The model under review builds one solid part; all positions refer to its coordinate system, in mm. A direction names the side the tool comes from. Round coordinates to 2 decimals unless told otherwise and drop trailing zeros. Write each loop counter-clockwise with the first axis right and the second up, starting at its lowest first coordinate (ties: lowest second). Pieces come first, ordered by that corner, then holes. Notation, with made-up numbers: (45, 88) - (80, 88) arc R11 ccw to (80, 97) - close; hole circle Ø10 at (37.25, 76). An arc over 180 degrees is marked (long way). Write each question's results on one line, items separated by ' | '.
```python
from build123d import *

# Parameters (mm, degrees)
F1_DEPTH      = 8
F1_DEPTH_BACK = 15
F0_R          = 3
F2_DEPTH      = 5
F3_R          = 2
F4_DEPTH      = 25


with BuildPart() as f1:
    # F0 (on Top) → F1 (new body, two sides)
    with BuildSketch(Plane.XY) as f1_sk:
        with BuildLine():
            Line((0, -25), (-25, 0))
            ThreePointArc((-25, 0), (-17.67767, -17.67767), (0, -25))
        make_face()
    extrude(amount=F1_DEPTH)
    extrude(f1_sk.sketch, amount=-F1_DEPTH_BACK)

    # F0 (on Top) → F2 (join)
    with BuildSketch(Plane.XY):
        with BuildLine():
            Line((-25, 0), (-30, 0))
            Line((-30, 0), (-30, -30))
            Line((-30, -30), (0, -30))
            Line((0, -30), (0, -25))
            ThreePointArc((0, -25), (-17.67767, -17.67767), (-25, 0))
        make_face()
        with Locations((-21.9205, -21.92012)):
            Circle(F0_R, mode=Mode.SUBTRACT)
    extrude(amount=F2_DEPTH)

    # F3 (on face) → F4 (cut)
    with BuildSketch(Plane(origin=(-12.5, -12.5, 0), x_dir=(-0.707107, 0.707107, 0), z_dir=(0.707107, 0.707107, 0))):
        with Locations((0, -9)):
            Circle(F3_R)
    extrude(amount=-F4_DEPTH, mode=Mode.SUBTRACT)


solid = f1.part
```
Q1. We need section D-D (x = -7). State the section outline as (y, z) points.
Evaluation:
outline: (-30, 0) - (-24, 0) - (-24, -15) - (-18, -15) - (-18, 8) - (-24, 8) - (-24, 5) - (-30, 5) - close
Q2. We need section C-C (z = -8). State the section outline as (x, y) points, plus the area to 3 significant figures.
Evaluation:
outline: (-25, 0) arc R25 ccw to (-18.86, -16.41) - (-13.72, -11.28) - close; (-16.41, -18.86) arc R25 ccw to (0, -25) - (-11.28, -13.72) - close | area: 153 mm^2
Q3. Insertion check: P1, Ø1, axis at x = -7.5, z = -12.5, coming from the +Y side; P2, Ø2, axis at y = -4.5, z = -3.5, coming from the -X side; P3, Ø1.5, axis at x = -4, z = -11.5, coming from the +Y side. Each pin has a flat end and moves straight along its axis. Give the tip position at first contact, or say it passes through.
Evaluation:
P1: stops at y = -17 | P2: stops at x = -24.75 | P3: stops at y = -20.25
Q4. Tool access review of faces 1 (the flat face through (-14, -14, -15)), 2 (the flat face through (-22, -18, 5)), 3 (the cylindrical face through (-17.871, -17.482, -5.728)): name each direction out of +Z, -Z, +X, -X, +Y, -Y from which nothing blocks a thin tool from reaching the whole face with its end or side.
Evaluation:
face 1: -Z, +X, -X, +Y, -Y | face 2: +Z, -X, -Y | face 3: -Z, -X, -Y
Q5. For probe 1 along Z at (x, y) = (-15, -24); probe 2 along Y at (x, z) = (-4.5, 6); probe 3 along X at (y, z) = (-22, 0.5), list the stretches that pass through material, from the lowest coordinate up.
Evaluation:
probe 1: z = 0 to 5 | probe 2: y = -24.59 to -20.5 | probe 3: x = -30 to -24.92, -18.92 to -3
Q6. The part is to be moulded in two halves that separate along X. For faces 4 (the flat face through (-22, -18, 0)), 5 (the cylindrical face through (-17.871, -17.482, 6.521)), 6 (the cylindrical face through (-15, -15, -7)), say which applies: released by +X, released by -X, zero draft, split by the parting line, or undercut.
Evaluation:
face 4: zero draft | face 5: released by -X | face 6: undercut
Q7. We need section A-A (x = -19.5). State the section outline as (y, z) points.
Evaluation:
outline: (-30, 0) - (-23.69, 0) - (-23.69, 5) - (-30, 5) - close; (-20.15, 0) - (-15.64, 0) - (-15.64, -15) - (-5.5, -15) - (-5.5, 8) - (-15.64, 8) - (-15.64, 5) - (-20.15, 5) - close
Q8. We need section B-B (y = -24). State the section outline as (x, z) points, plus the area to 3 significant figures.
Evaluation:
outline: (-30, 0) - (-24.08, 0) - (-24.08, 5) - (-30, 5) - close; (-19.76, 0) - (-7, 0) - (-7, -15) - (-1, -15) - (-1, 8) - (-7, 8) - (-7, 5) - (-19.76, 5) - close | area: 231 mm^2
